from build123d import *

# Parameters (mm, degrees)
PAD_DEPTH           = 1.5
POCKET_DEPTH        = 5
POCKET001_DEPTH     = 5
LINEARPATTERN_COUNT = 8
LINEARPATTERN_PITCH = 3.857143
SKETCH003_R         = 1.375
POCKET002_DEPTH     = 5


with BuildPart() as part:
    # Sketch → Pad (new body)
    with BuildSketch(Plane.XY):
        with BuildLine():
            Line((-43.5, 20), (43.5, 20))
            ThreePointArc((46.5, 17), (45.62132, 19.12132), (43.5, 20))
            Line((46.5, 17), (46.5, -17))
            ThreePointArc((43.5, -20), (45.62132, -19.12132), (46.5, -17))
            Line((43.5, -20), (-35, -20))
            ThreePointArc((-38, -17), (-37.12132, -19.12132), (-35, -20))
            Line((-38, -9.5), (-38, -17))
            Line((-43.5, -9.5), (-38, -9.5))
            ThreePointArc((-46.5, -6.5), (-45.62132, -8.62132), (-43.5, -9.5))
            Line((-46.5, 17), (-46.5, -6.5))
            ThreePointArc((-43.5, 20), (-45.62132, 19.12132), (-46.5, 17))
        make_face()
    extrude(amount=PAD_DEPTH)

    # Sketch001 (on Face13 of Pad) → Pocket (cut)
    with BuildSketch(Plane.XY.offset(1.5)):
        with BuildLine():
            Line((2.5, 9.5), (34.5, 9.5))
            ThreePointArc((36, 8), (35.56066, 9.06066), (34.5, 9.5))
            Line((36, 8), (36, -12))
            ThreePointArc((34.5, -13.5), (35.56066, -13.06066), (36, -12))
            Line((34.5, -13.5), (2.5, -13.5))
            ThreePointArc((1, -12), (1.43934, -13.06066), (2.5, -13.5))
            Line((1, -12), (1, 8))
            ThreePointArc((2.5, 9.5), (1.43934, 9.06066), (1, 8))
        make_face()
    extrude(amount=-POCKET_DEPTH, mode=Mode.SUBTRACT)

    # Sketch002 (on Face5 of Pocket) → Pocket001 (cut)
    with BuildSketch(Plane.XY.offset(1.5)):
        with BuildLine():
            ThreePointArc((-30.8, 12.3), (-32, 13.5), (-33.2, 12.3))
            Line((-33.2, 12.3), (-33.2, -12.3))
            ThreePointArc((-33.2, -12.3), (-32, -13.5), (-30.8, -12.3))
            Line((-30.8, -12.3), (-30.8, 12.3))
        make_face()
    pocket001 = extrude(amount=-POCKET001_DEPTH, mode=Mode.SUBTRACT)

    # LinearPattern: Pocket001 ×8
    with Locations(*[(i * LINEARPATTERN_PITCH, 0, 0) for i in range(1, LINEARPATTERN_COUNT)]):
        add(pocket001, mode=Mode.SUBTRACT)

    # Sketch003 (on Face5 of LinearPattern) → Pocket002 (cut)
    with BuildSketch(Plane.XY.offset(1.5)):
        with Locations((42.375, 15.86)):
            Circle(SKETCH003_R)
        with Locations((-42.375, 15.86)):
            Circle(SKETCH003_R)
        with Locations((42.375, -15.86)):
            Circle(SKETCH003_R)
        with Locations((-42.375, -5.36)):
            Circle(SKETCH003_R)
    extrude(amount=-POCKET002_DEPTH, mode=Mode.SUBTRACT)


solid = part.part
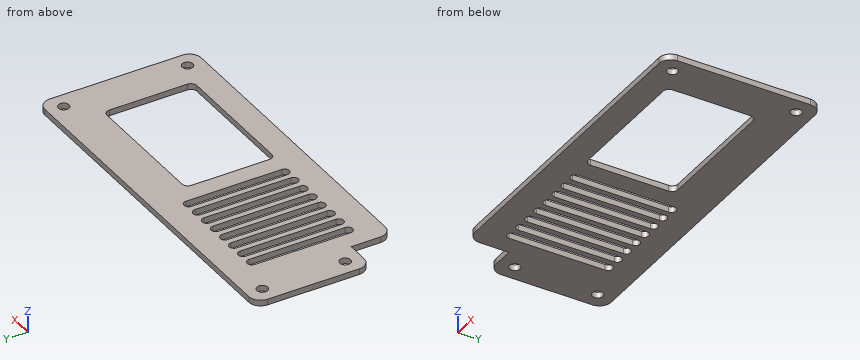
Input: part model. Units: mm. Frame: model coordinates. Give positions to 0.01 mm unless a question says otherwise; leave off trailing zeros. Order: outer loops, then holes, each group sorted by start corner. A loop starts at its lowest first (then second) coordinate and runs counter-clockwise, first axis right, second up. Notation, with made-up numbers: (6.5, 70) - (40.5, 70) arc R15 cw to (40.5, 79) - close; hole circle Ø2 at (9, -22.5). An arc over 180 degrees is marked (long way). Answer as a JSON object with one key per item and string values. Group by question number.
Q1. Cut plane C-C, the plane y = -15.86. Output: boundary loops of the cut face in (x, z).
Q2. Cut plane A-A, the plane x = 6.5. Output: boundary loops of the cut face in (y, z), then the cut area to 3 significant figures.
Q3. Line query: probe 1 along Y at (x, z) = (-43, 0.75); probe 2 along X at (y, z) = (15, 0.5); probe 3 along Y at (x, z) = (-5, 1.3). Output: solid intervals per line, ascending.
Q4. Cut plane B-B, the plane y = 15.86. Output: boundary loops of the cut face in (x, z), then the cut area to 3 significant figures.
Q5. First-contact query: pin 1 Ø0.8 at (y, z) = (-11.5, 1) entering from -X. Flat tip, straight axial feed; report the tip coordinate or a pass-through.
Q6. Cut plane D-D, the plane z = 0.4. Count the separate pieces of the cut face and the enclosed holes in it, then the cut area to 3 significant figures.
Results:
{
 "1": {"outline": "(-38, 0) - (41, 0) - (41, 1.5) - (-38, 1.5) - close; (43.75, 0) - (46.5, 0) - (46.5, 1.5) - (43.75, 1.5) - close"},
 "2": {"outline": "(-20, 0) - (-13.5, 0) - (-13.5, 1.5) - (-20, 1.5) - close; (9.5, 0) - (20, 0) - (20, 1.5) - (9.5, 1.5) - close", "area": "25.5 mm^2"},
 "3": {"probe 1": "-9.5 to -6.58, -4.14 to 14.64, 17.08 to 20", "probe 2": "-46.5 to -43.45, -41.3 to 41.3, 43.45 to 46.5", "probe 3": "-20 to -13.5, 13.5 to 20"},
 "4": {"outline": "(-46.5, 0) - (-43.75, 0) - (-43.75, 1.5) - (-46.5, 1.5) - close; (-41, 0) - (41, 0) - (41, 1.5) - (-41, 1.5) - close; (43.75, 0) - (46.5, 0) - (46.5, 1.5) - (43.75, 1.5) - close", "area": "131 mm^2"},
 "5": {"pin 1": "x = -38"},
 "6": {"separate pieces": "1", "enclosed holes": "13", "area": "2,290 mm^2"}
}
